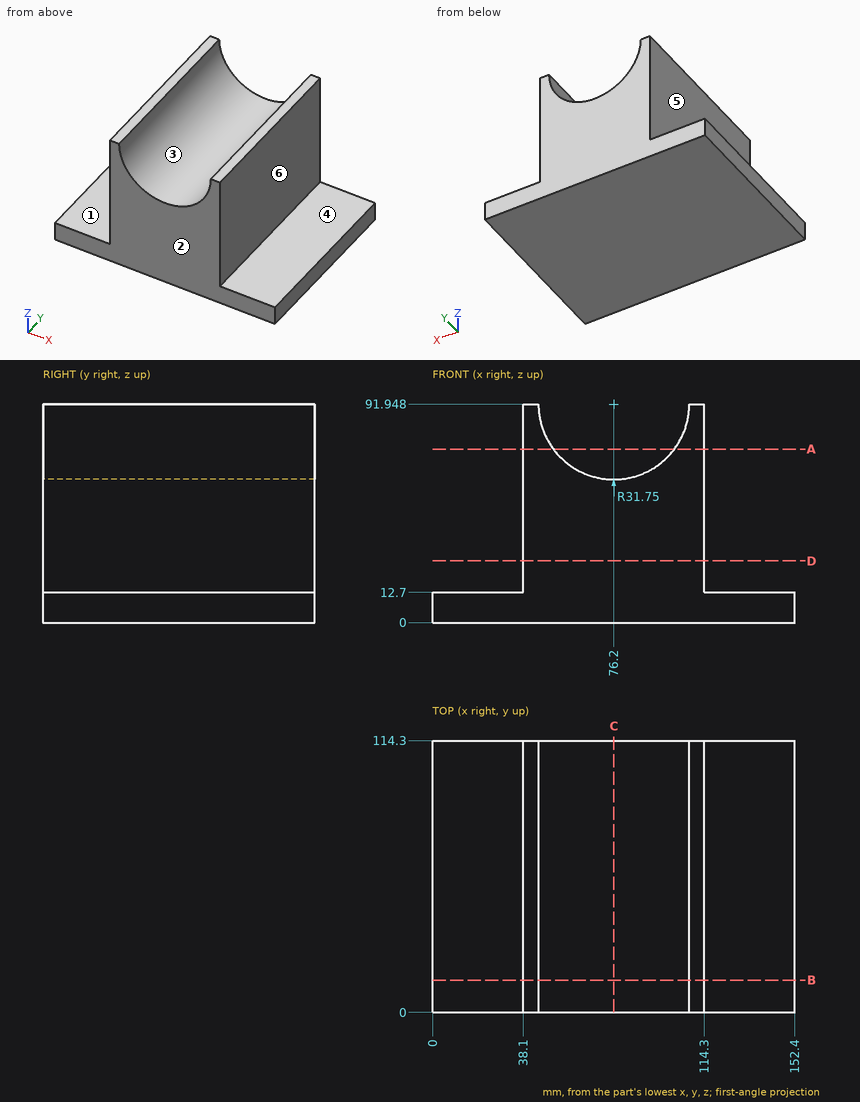
Part print with two shaded views. Sizes in mm from the minimum x, y, z corner. A direction names the side the tool comes from. Give positions to 0.01 mm unless a question says otherwise; leave off trailing zeros. Write each loop counter-clockwise with the first axis right and the second up, starting at its lowest first coordinate (ties: lowest second). Pieces come first, ordered by that corner, then holes.
1) Pin check, flat tips, straight feed: pin 1 (24 mm diameter, centred on y = 34, z = 64, fed in from -X); pin 2 (1.5 mm diameter, centred on x = 25.5, y = 85.5, fed in from +Z); pin 3 (24 mm diameter, centred on y = 82, z = 53, fed in from +X). Stop position of each tip, or through.
Resolved:
pin 1: stops at x = 38.1
pin 2: stops at z = 12.7
pin 3: stops at x = 114.3
2) Cut at C-C on x = 76.2. Write the cut outline in (y, z), then the cut area to 3 significant figures.
Resolved:
outline: (0, 0) - (114.3, 0) - (114.3, 60.2) - (0, 60.2) - close
area: 6,880 mm2
3) Cut at A-A on z = 73. Write the cut outline in (x, y).
Resolved:
outline: (38.1, 0) - (50.72, 0) - (50.72, 114.3) - (38.1, 114.3) - close; (101.68, 0) - (114.3, 0) - (114.3, 114.3) - (101.68, 114.3) - close
4) Cut at B-B on y = 13.5. Write the cut outline in (x, z).
Resolved:
outline: (0, 0) - (152.4, 0) - (152.4, 12.7) - (114.3, 12.7) - (114.3, 91.95) - (107.95, 91.95) arc R31.75 cw to (44.45, 91.95) - (38.1, 91.95) - (38.1, 12.7) - (0, 12.7) - close
5) Which spindle directions (+Z, -Z, +X, -X, +Y, -Y) get a long thin tool onto all of the face, cutting with end or side? Do the marked faces 1 and 2. Say none if no direction does.
Resolved:
face 1: +Z, -X, +Y, -Y
face 2: +Z, -Z, +X, -X, -Y
6) Probe L1, parallel to Z at x = 17, y = 86; L2, parallel to X at y = 28, z = 23; L3, parallel to X at y = 89.5, z = 67. List the from-to ranges inside material, lowest first.
Resolved:
L1: z = 0 to 12.7
L2: x = 38.1 to 114.3
L3: x = 38.1 to 56.56, 95.84 to 114.3
7) Cut at D-D on z = 26. Write the cut outline in (x, y), then the cut area to 3 significant figures.
Resolved:
outline: (38.1, 0) - (114.3, 0) - (114.3, 114.3) - (38.1, 114.3) - close
area: 8,710 mm2
8) Two-plate mould, pull along X, no slides. Class the marked faces 3, 4, 5 and 6: released by +X, released by -X, zero draft, split by the parting line, or undercut.
Resolved:
face 3: undercut
face 4: zero draft
face 5: released by -X
face 6: released by +X
